Job drawing, mm, ordinate dimensions from the low corner. One solid piece. A direction names the side the tool comes from. Give positions to 0.01 mm unless a question says otherwise; leave off trailing zeros. Loops run counter-clockwise (first coordinate to the right, second up) from the corner with the lowest first, then second, coordinate; pieces in that order, holes last. Notation, with made-up numbers: (64, 61) -> (91, 61) arc R13 ccw to (91, 81) -> close; hole circle Ø1 at (83.25, 35). An arc over 180 degrees is marked (long way). Use one line per item in the form item = value.
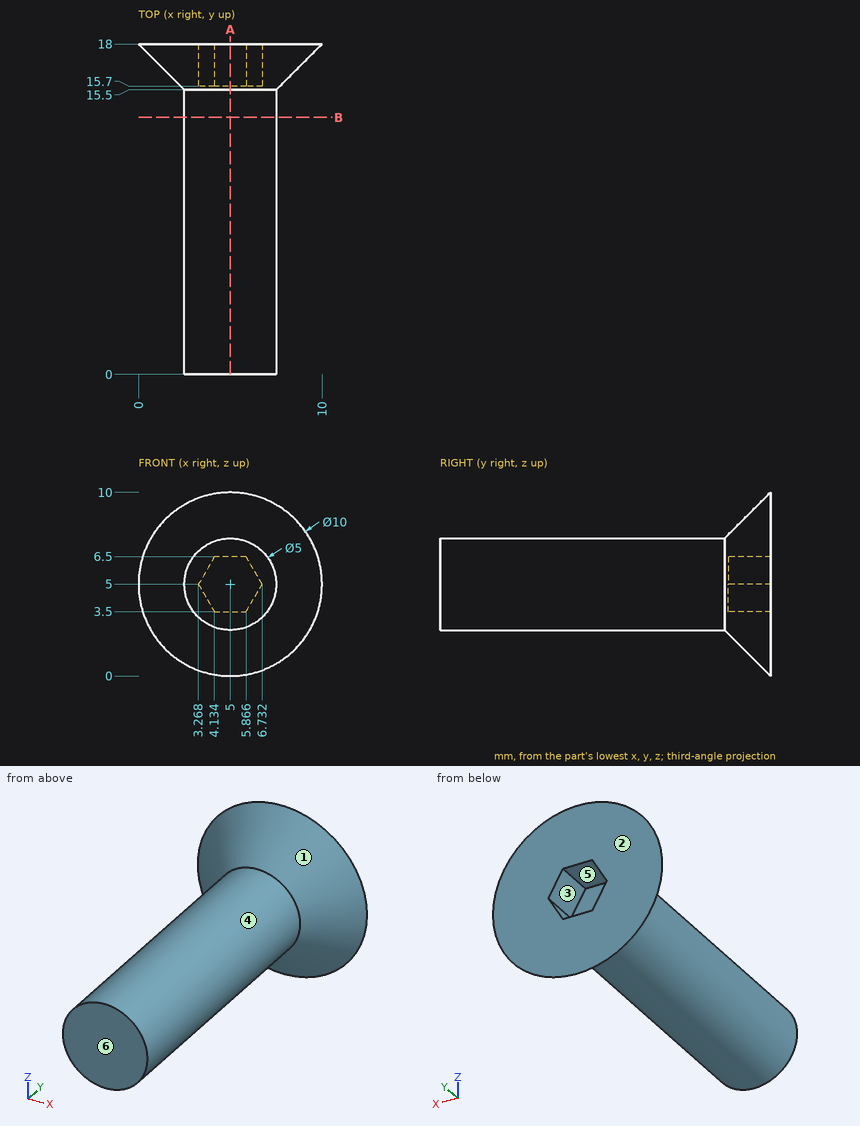
1. Mould opens along X. For the marked faces 1, 2 and 3 say: pulls with the +X half, pulls with the -X half, needs draft (parallel to the pull), parting line crosses it, or undercut.
Result sheet:
face_1 = parting line crosses it
face_2 = needs draft
face_3 = undercut
2. Tool access for the marked faces 4, 5 and 6: list every direction of +Z, -Z, +X, -X, +Y, -Y with a clear straight run to the whole face (end or side of a thin tool).
Result sheet:
face_4 = -Y
face_5 = +Y
face_6 = +Z, -Z, +X, -X, -Y
3. Drill centre lines: line 1 (Y direction, x = 5.75, z = 6); line 2 (Z direction, x = 5.5, y = 3.25); line 3 (Z direction, x = 6.75, y = 12.5) (1 decimal). Where is each one in solid material? Low to high.
Result sheet:
line_1 = 0 to 15.7
line_2 = 2.55 to 7.45
line_3 = 3.2 to 6.8
4. Cut at A-A, the plane x = 5. Write the cut outline in (y, z).
Result sheet:
outline = (0, 2.5) -> (15.5, 2.5) -> (18, 0) -> (18, 3.5) -> (15.7, 3.5) -> (15.7, 6.5) -> (18, 6.5) -> (18, 10) -> (15.5, 7.5) -> (0, 7.5) -> close
5. Drop flat-ended pins along their axis: P1, Ø1.4, axis at x = 5, y = 17, coming from the +Z side; P2, Ø5, axis at y = 16, z = 8, coming from the -X side; P3, Ø1.4, axis at x = 5, y = 16.5, coming from the -Z side. Give the stop position or say it passes through.
Result sheet:
P1 = 9.7
P2 = 0.23
P3 = 0.8
6. Cut at B-B, the plane y = 14. Write the cut outline in (x, z).
Result sheet:
outline = circle Ø5 at (5, 5)
